The drawing under review shows one solid part. Ordinate dimensions are in mm from its lowest x, y, z. A direction names the side the tool comes from. Round coordinates to 2 decimals unless told otherwise and drop trailing zeros. Write each loop counter-clockwise with the first axis right and the second up, starting at its lowest first coordinate (ties: lowest second). Pieces come first, ordered by that corner, then holes. Notation, with made-up numbers: (56, 29.25) -> (79, 29.25) arc R27 ccw to (79, 68.25) -> close; hole circle Ø3 at (55, -21). An arc over 180 degrees is marked (long way). Answer in a Markdown table with one row per item.
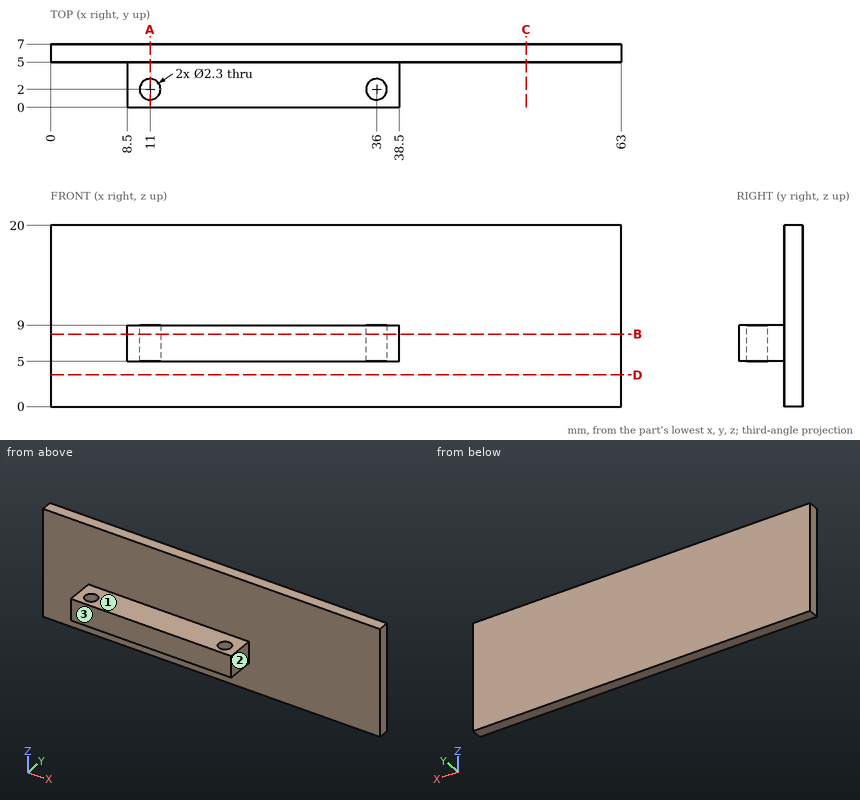
1) For line 1 (Y direction, x = 11, z = 6.05); line 2 (Z direction, x = 27, y = 4.25); line 3 (Y direction, x = 56, z = 8.5), list the stretches that pass through material, from the lowest coordinate up. Write a range as [from, to].
Solved:
| item | result |
|---|---|
| line 1 | [0, 0.85], [3.15, 7] |
| line 2 | [5, 9] |
| line 3 | [5, 7] |
2) For the marked faces 1, 2 and 3, list the 3-axis set-ups (+Z, -Z, +X, -X, +Y, -Y) from which the entire face can be reached by the end or side of a thin tool; tool diameter is ignored.
Solved:
| item | result |
|---|---|
| face 1 | +Z, +X, -X, -Y |
| face 2 | +Z, -Z, +X, -Y |
| face 3 | +Z, -Z, +X, -X, -Y |
3) Consider section C-C on x = 52.5. State the section outline as (y, z) points.
Solved:
| item | result |
|---|---|
| outline | (5, 0) -> (7, 0) -> (7, 20) -> (5, 20) -> close |
4) Consider section B-B on z = 8. State the section outline as (x, y) points, then the cut area to 3 significant figures.
Solved:
| item | result |
|---|---|
| outline | (0, 5) -> (8.5, 5) -> (8.5, 0) -> (38.5, 0) -> (38.5, 5) -> (63, 5) -> (63, 7) -> (0, 7) -> close; hole circle Ø2.3 at (11, 2); hole circle Ø2.3 at (36, 2) |
| area | 268 mm² |
5) Consider section D-D on z = 3.5. State the section outline as (x, y) points.
Solved:
| item | result |
|---|---|
| outline | (0, 5) -> (63, 5) -> (63, 7) -> (0, 7) -> close |
6) Clearance check with flat-ended pins moving along their axes: pin 1 Ø1.5 at (x, y) = (18, 4.5) entering from +Z; pin 2 Ø1 at (y, z) = (3, 15.5) entering from +X; pin 3 Ø10 at (x, z) = (44, 6.5) entering from -Y; pin 4 Ø2 at (y, z) = (3.5, 6.5) entering from +X. State where each tip first meets the part, or that it passes through.
Solved:
| item | result |
|---|---|
| pin 1 | z = 20 |
| pin 2 | through |
| pin 3 | y = 5 |
| pin 4 | x = 38.5 |
7) Consider section A-A on x = 11. State the section outline as (y, z) points.
Solved:
| item | result |
|---|---|
| outline | (0, 5) -> (0.85, 5) -> (0.85, 9) -> (0, 9) -> close; (3.15, 5) -> (5, 5) -> (5, 0) -> (7, 0) -> (7, 20) -> (5, 20) -> (5, 9) -> (3.15, 9) -> close |
